Check sheet for the modelled part. Datum: model origin and axes. Units: mm. Face numbers are marked on the shaded views. A direction names the side the tool comes from. Round coordinates to 2 decimals unless told otherwise and drop trailing zeros. Order: outer loops, then holes, each group sorted by start corner. A loop starts at its lowest first (then second) coordinate and runs counter-clockwise, first axis right, second up. Notation, with made-up numbers: (-19.5, -5) -> (35.5, -5) arc R17 ccw to (35.5, 11) -> close; hole circle Ø9 at (13.5, 77). An arc over 180 degrees is marked (long way). Use CSV: the item, a comma, the result in double quotes.
```python
from build123d import *

# Parameters (mm, degrees)
BOSS_EXTRUDE2_DEPTH = 16
BOSS_EXTRUDE3_DEPTH = 16
FILLET9_R           = 0.5
BOSS_EXTRUDE4_DEPTH = 1
FILLET10_R          = 1


with BuildPart() as part:
    # Sketch5 → Boss-Extrude2 (new body)
    with BuildSketch(Plane(origin=(4.228476288, 0, 0), x_dir=(1, 0, 0), z_dir=(0, 0, 1))):
        with BuildLine():
            Line((-3.568997542, 0.452866188), (-2.852532713, 0.71363806))
            ThreePointArc((-2.852532713, 0.71363806), (-5.778476288, 0), (-2.852532713, -0.71363806))
            Line((-2.852532713, -0.71363806), (-3.568997542, -0.452866188))
            ThreePointArc((-3.568997542, -0.452866188), (-5.028476288, 0), (-3.568997542, 0.452866188))
        make_face()
    extrude(amount=BOSS_EXTRUDE2_DEPTH)

    # Sketch6 → Boss-Extrude3 (add)
    with BuildSketch(Plane.XY.offset(16)):
        Polygon((-8.907406692, 6.008719055), (-8.407406692, 6.874744459), (0.252847346, 1.874744459), (1.327591805, 0.8), (0.114359354, 0.8), align=None)
        Polygon((0.252847346, -1.874744459), (1.327591805, -0.8), (0.114359354, -0.8), (-8.907406692, -6.008719055), (-8.407406692, -6.874744459), align=None)
    extrude(amount=-BOSS_EXTRUDE3_DEPTH)

    # Fillet9
    fillet9_edges = [part.edges().sort_by_distance(p)[0] for p in [
        (0.659478746, -0.452866188, 8),
        (0.659478746, 0.452866188, 8),
    ]]
    fillet(fillet9_edges, radius=FILLET9_R)

    # Sketch7 → Boss-Extrude4 (add)
    with BuildSketch(Plane(origin=(0, 0, 0), x_dir=(-1, 0, 0), z_dir=(0, 0, -1))):
        Polygon((8.407406692, 6.874744459), (4.943305077, 4.874744459), (3.443305077, 7.47282067), (6.907406692, 9.47282067), align=None)
        Polygon((6.907406692, -9.47282067), (3.443305077, -7.47282067), (4.943305077, -4.874744459), (8.407406692, -6.874744459), align=None)
        Polygon((8.907406692, 6.008719055), (7.175355885, 5.008719055), (7.675355885, 4.142693652), (9.407406692, 5.142693652), align=None)
        Polygon((9.407406692, -5.142693652), (7.675355885, -4.142693652), (7.175355885, -5.008719055), (8.907406692, -6.008719055), align=None)
    extrude(amount=-BOSS_EXTRUDE4_DEPTH)

    # Fillet10
    fillet10_edges = [part.edges().sort_by_distance(p)[0] for p in [
        (-0.799734012, 1.327752051, 8),
        (-0.799734012, -1.327752051, 8),
    ]]
    fillet(fillet10_edges, radius=FILLET10_R)


solid = part.part
```
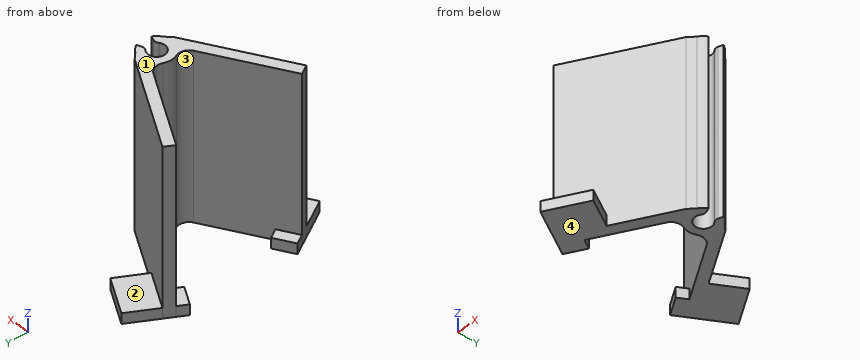
Q1. Sectioned sample at D-D, the plane y = 0. Enter the section's corners in (x, z).
Result sheet:
outline,"(-1.55, 0) -> (-0.8, 0) -> (-0.8, 16) -> (-1.55, 16) -> close"
Q2. Mould release check, pull along Y, two halves, no side actions. Record for the marked faces 3 and 4: pulls with the +Y half, pulls with the -Y half, needs draft (parallel to the pull), parting line crosses it, or undercut.
Result sheet:
face 3,"undercut"
face 4,"needs draft"
Q3. Sectioned sample at B-B, the plane z = 11.5. Enter the section's corners in (x, y).
Result sheet:
outline,"(-8.91, -6.01) -> (-8.41, -6.87) -> (0.25, -1.87) -> (0.8, -1.33) arc R1.55 ccw to (1.38, -0.71) -> (0.96, -0.56) arc R0.5 ccw to (0.49, -0.64) arc R0.8 cw (long way) to (0.49, 0.64) arc R0.5 ccw to (0.96, 0.56) -> (1.38, 0.71) arc R1.55 ccw to (0.8, 1.33) -> (0.25, 1.87) -> (-8.41, 6.87) -> (-8.91, 6.01) -> (-1.82, 1.92) arc R1 cw to (-1.41, 0.64) arc R1.55 ccw to (-1.41, -0.64) arc R1 cw to (-1.82, -1.92) -> close"
Q4. Sectioned sample at C-C, the plane x = 0. Enter the section's corners in (y, z).
Result sheet:
outline,"(-2.02, 0) -> (-0.8, 0) -> (-0.8, 16) -> (-2.02, 16) -> close; (0.8, 0) -> (2.02, 0) -> (2.02, 16) -> (0.8, 16) -> close"
Q5. Go/stop test with flat-tipped pins: pin 1 (4 mm diameter, centred on y = 2, z = 6, fed in from -X); pin 2 (2 mm diameter, centred on y = -7.5, z = 14, fed in from -X); pin 3 (1.4 mm diameter, centred on x = -5.5, y = -7, fed in from +Z); pin 4 (5 mm diameter, centred on x = -3, y = -6, fed in from +Z). Record where each tip stops, or that it passes through.
Result sheet:
pin 1,"stops at x = -5.43"
pin 2,"stops at x = -8.62"
pin 3,"stops at z = 1"
pin 4,"stops at z = 16"
Q6. Scan lines: L1, parallel to Y at x = -4.25, z = 3; L2, parallel to Y at x = -8.75, z = 7; L3, parallel to Z at x = -7.5, y = -5. Record each from-to range of solid material in increasing order.
Result sheet:
L1,"y = -4.47 to -3.32, 3.32 to 4.47"
L2,"y = -6.28 to -5.92, 5.92 to 6.28"
L3,"z = 0 to 1"
Q7. Sectioned sample at A-A, the plane x = -2.75. Enter the section's corners in (y, z).
Result sheet:
outline,"(-3.61, 0) -> (-2.45, 0) -> (-2.45, 16) -> (-3.61, 16) -> close; (2.45, 0) -> (3.61, 0) -> (3.61, 16) -> (2.45, 16) -> close"
Q8. Access from +Z, -Z, +X, -X, +Y, -Y to the whole of each face (thin tool, end or side, straight path). Record for the marked faces 1 and 2.
Result sheet:
face 1,"+Z, +X, -X, +Y, -Y"
face 2,"+Z, +X, +Y"
